Could you check a few things on this model? Use its own coordinates, in mm. A direction names the side the tool comes from. Coordinates: 2 decimals unless noted, no trailing zeros. Order: outer loops, then holes, each group sorted by start corner. A loop starts at its lowest first (then second) coordinate and runs counter-clockwise, first axis right, second up. Notation, with made-up numbers: (57.25, 72) - (87.25, 72) arc R14 ccw to (87.25, 98) - close; hole circle Ø10 at (69.5, 40). An arc over 180 degrees is marked (long way). Answer as a JSON object with one key per item and string values. Group by question number.
(1) We'd pull the mould along Z, two halves only. Please class faces 3 (the flat face through (0, -6, 22)), 4 (the flat face through (-228, -6, 0)), 5 (the flat face through (-170, -5, 15)), 6 (the cylindrical face through (-270.604, -2.465, 15.193)): pulls with the +Z half, pulls with the -Z half, needs draft (parallel to the pull), parting line crosses it, or undercut.
(2) Will these pins go through, and if not, where does the flat tip stop? P1, Ø8.5, axis at x = -275, z = 15, coming from the -Y side; P2, Ø10, axis at x = -275, z = 15, coming from the -Y side.
(3) Imagine slicing it at A-A, the plane z = 15. Write out the boundary of the cut face in (x, y) (3 decimals).
(4) Imagine slicing it at C-C, the plane x = -275. Write out the boundary of the cut face in (y, z) (3 decimals), and give its area (3 significant figures).
(5) Please list where these lines run through material, in increasing order: probe 1 along Z at (x, y) = (-20, -6.5); probe 2 along Z at (x, y) = (-175, -2.35); probe 3 along X at (y, z) = (-5, 23).
(6) Imagine slicing it at B-B, the plane y = -10.5. Write out the boundary of the cut face in (x, z) (3 decimals).
(7) Which directions (+Z, -Z, +X, -X, +Y, -Y) give clear straight access to the entire face, cutting with the end or side of a thin tool? Please do faces 1 (the cylindrical face through (-179.197, -2.465, 16.322)), 2 (the flat face through (-270, -5, 15)).
from build123d import *

# Parameters (mm, degrees)
F0_W           = 450
F0_H           = 44
F1_DEPTH       = 13
F3_D           = 5
F4_D           = 8.8
F4_CBORE_D     = 14.25
F4_CBORE_DEPTH = 8


with BuildPart() as f1:
    # F0 (on Front) → F1 (new body)
    with BuildSketch(Plane.XZ):
        with Locations((-225, 22)):
            Rectangle(F0_W, F0_H)
    extrude(amount=F1_DEPTH)

    # F3 (through all)
    with Locations(Plane.XZ.offset(13)):
        with Locations((-430, 22), (-20, 22)):
            Hole(F3_D / 2)

    # F4 (through all)
    with Locations(Plane.XZ.offset(13)):
        with Locations((-275, 15), (-175, 15)):
            CounterBoreHole(F4_D / 2, F4_CBORE_D / 2, F4_CBORE_DEPTH)


solid = f1.part
Result set:
{
 "1": {"face 3": "needs draft", "face 4": "pulls with the -Z half", "face 5": "undercut", "face 6": "undercut"},
 "2": {"P1": "passes through", "P2": "stops at y = -5"},
 "3": {"outline": "(-450, -13) - (-282.125, -13) - (-282.125, -5) - (-279.4, -5) - (-279.4, 0) - (-450, 0) - close; (-270.6, -5) - (-267.875, -5) - (-267.875, -13) - (-182.125, -13) - (-182.125, -5) - (-179.4, -5) - (-179.4, 0) - (-270.6, 0) - close; (-170.6, -5) - (-167.875, -5) - (-167.875, -13) - (0, -13) - (0, 0) - (-170.6, 0) - close"},
 "4": {"outline": "(-13, 0) - (0, 0) - (0, 10.6) - (-5, 10.6) - (-5, 7.875) - (-13, 7.875) - close; (-13, 22.125) - (-5, 22.125) - (-5, 19.4) - (0, 19.4) - (0, 44) - (-13, 44) - close", "area": "414 mm^2"},
 "5": {"probe 1": "z = 0 to 19.5, 24.5 to 44", "probe 2": "z = 0 to 10.6, 19.4 to 44", "probe 3": "x = -450 to -432.29, -427.71 to -22.29, -17.71 to 0"},
 "6": {"outline": "(-450, 0) - (0, 0) - (0, 44) - (-450, 44) - close; hole circle Ø5 at (-430, 22); hole circle Ø14.25 at (-275, 15); hole circle Ø14.25 at (-175, 15); hole circle Ø5 at (-20, 22)"},
 "7": {"face 1": "+Y, -Y", "face 2": "-Y"}
}
